Model file for the job. Use its own axes, mm. A direction names the side the tool comes from. Coordinates: 2 decimals unless noted, no trailing zeros. Write each loop counter-clockwise with the first axis right and the second up, starting at its lowest first coordinate (ties: lowest second). Pieces come first, ordered by that corner, then holes.
Q1. Band-saw the part on A-A, the plane z = 0. Write the cut outline in (x, y).
Q2. Drill centre lines: probe 1 along Y at (x, z) = (-3, 1); probe 2 along Z at (x, y) = (1.75, 4.25); probe 3 along X at (y, z) = (2.5, 0). Where is each one in solid material? Low to high.
Q3. Band-saw the part on C-C, the plane y = 2.25. Write the cut outline in (x, z).
Q4. Which spindle directions (+Z, -Z, +X, -X, +Y, -Y) get a long thin tool onto all of the face, cutting with end or side? Do faces 4 (the flat face through (-1.6, 4.4, -2)), 5 (the cylindrical face through (-3.593, 2.328, 1.869)). Say none if no direction does.
Q5. Band-saw the part on B-B, the plane x = 0. Write the cut outline in (y, z).
Q6. Pin check, flat tips, straight feed: P1, Ø0.8, axis at x = -1, z = -1.5, coming from the -Y side; P2, Ø1, axis at y = 0.5, z = -4, coming from the -X side; P3, Ø1.5, axis at x = 0.5, z = 0.5, coming from the +Y side. Stop position of each tip, or through.
Q7. Pull direction X, two halves, no side cores. Call faces 1 (the cylindrical face through (0.194, 0.246, 4.596)), 2 (the flat face through (0, 4.1, 0)), 3 (the flat face through (-1.6, 4.4, 2.1)): released by +X, released by -X, zero draft, split by the parting line, or undercut.
from build123d import *

# Parameters (mm, degrees)
SKETCH1_R                   = 4.05
BASE_EXTRUSION_DEPTH        = 4.2
SKETCH2_W                   = 3
SKETCH2_H                   = 4
WINDOW_DEPTH                = 0.1
WINDOW_BUMPS_DEPTH          = 0.2
WINDOW_BUMPS_CHAMFERS_SIZE  = 0.2
SKETCH3_R                   = 4.6
FLANGE_DEPTH                = 0.5
SKETCH5_W                   = 1.15
SKETCH5_H                   = 1
HORIZONTAL_FLANGE_TAB_DEPTH = 0.5
ROUNDS_AND_FILLETS_R        = 0.25
SKETCH4_R                   = 0.25
LEADS_DEPTH                 = 13.2


with BuildPart() as part:
    # Sketch1 → Base Extrusion (new body)
    with BuildSketch(Plane(origin=(0, 0, 0), x_dir=(1, 0, 0), z_dir=(0, 1, 0))):
        with Locations(Location((0, 0, 0), (0, 0, 270))):
            Circle(SKETCH1_R)
    extrude(amount=BASE_EXTRUSION_DEPTH)

    # Sketch2 → Window (cut)
    with BuildSketch(Plane(origin=(0, 4.2, 0), x_dir=(1, 0, 0), z_dir=(0, 1, 0))):
        Rectangle(SKETCH2_W, SKETCH2_H)
    extrude(amount=-WINDOW_DEPTH, mode=Mode.SUBTRACT)

    # Sketch6 → Window Bumps (add)
    with BuildSketch(Plane(origin=(0, 4.2, 0), x_dir=(1, 0, 0), z_dir=(0, 1, 0))):
        with BuildLine():
            Line((-0.75, 2), (-1.5, 1.25))
            ThreePointArc((-1.5, 1.25), (-2.030330086, 2.530330086), (-0.75, 2))
        make_face()
        with BuildLine():
            Line((0.75, 2), (1.5, 1.25))
            ThreePointArc((1.5, 1.25), (2.030330086, 2.530330086), (0.75, 2))
        make_face()
        with BuildLine():
            Line((1.5, -1.25), (0.75, -2))
            ThreePointArc((0.75, -2), (2.030330086, -2.530330086), (1.5, -1.25))
        make_face()
        with BuildLine():
            Line((-1.5, -1.25), (-0.75, -2))
            ThreePointArc((-0.75, -2), (-2.030330086, -2.530330086), (-1.5, -1.25))
        make_face()
    extrude(amount=WINDOW_BUMPS_DEPTH)

    # Window Bumps Chamfers
    window_bumps_chamfers_edges = [part.edges().sort_by_distance(p)[0] for p in [
        (-2.030330086, 4.4, 2.530330086),
        (2.030330086, 4.4, 2.530330086),
        (2.030330086, 4.4, -2.530330086),
        (-2.030330086, 4.4, -2.530330086),
        (-1.125, 4.4, 1.625),
        (1.125, 4.4, 1.625),
        (1.125, 4.4, -1.625),
        (-1.125, 4.4, -1.625),
    ]]
    chamfer(window_bumps_chamfers_edges, length=WINDOW_BUMPS_CHAMFERS_SIZE - 0.0001)  # a hair under: the kernel refuses the full size

    # Sketch3 → Flange (add)
    with BuildSketch(Plane.XZ):
        with Locations(Location((0, 0, 0), (0, 0, 270))):
            Circle(SKETCH3_R)
    extrude(amount=-FLANGE_DEPTH)

    # Sketch5 → Horizontal Flange Tab (add)
    with BuildSketch(Plane.XZ):
        with Locations((0, -5.063921012)):
            Rectangle(SKETCH5_W, SKETCH5_H)
    extrude(amount=-HORIZONTAL_FLANGE_TAB_DEPTH)

    # Rounds and Fillets
    rounds_and_fillets_edges = [part.edges().sort_by_distance(p)[0] for p in [
        (0, 4.2, -4.05),
        (0, 0.5, -4.05),
        (-0.575, 0.25, -5.563921012),
        (0.575, 0.25, -5.563921012),
    ]]
    fillet(rounds_and_fillets_edges, radius=ROUNDS_AND_FILLETS_R)

    # Sketch4 → Leads (add)
    with BuildSketch(Plane.XZ):
        with Locations(Location((-1.796051224, -1.796051224, 0), (0, 0, 90))):
            Circle(SKETCH4_R)
        with Locations(Location((1.796051224, 1.796051224, 0), (0, 0, 90))):
            Circle(SKETCH4_R)
        with Locations(Location((-1.796051224, 1.796051224, 0), (0, 0, 90))):
            Circle(SKETCH4_R)
    extrude(amount=LEADS_DEPTH)

    # Leads Trim
    split(bisect_by=Plane(origin=(0, -2, 0), x_dir=(1, 0, 0), z_dir=(0, 1, 0)), keep=Keep.TOP)


solid = part.part
Answer sheet:
1. outline: (-4.6, 0) - (4.6, 0) - (4.6, 0.5) - (4.3, 0.5) arc R0.25 cw to (4.05, 0.75) - (4.05, 3.95) arc R0.25 ccw to (3.8, 4.2) - (1.5, 4.2) - (1.5, 4.1) - (-1.5, 4.1) - (-1.5, 4.2) - (-3.8, 4.2) arc R0.25 ccw to (-4.05, 3.95) - (-4.05, 0.75) arc R0.25 cw to (-4.3, 0.5) - (-4.6, 0.5) - close
2. probe 1: y = 0 to 4.2
2. probe 2: z = -2.65 to -1.35, 1.35 to 2.65
2. probe 3: x = -4.05 to 4.05
3. outline: circle Ø8.1 at (0, 0)
4. face 4: +Z, -Z, +X, -X, +Y
4. face 5: +Y
5. outline: (0, -5.56) - (0.5, -5.56) - (0.5, -4.3) arc R0.25 cw to (0.75, -4.05) - (3.95, -4.05) arc R0.25 ccw to (4.2, -3.8) - (4.2, -2) - (4.1, -2) - (4.1, 2) - (4.2, 2) - (4.2, 3.8) arc R0.25 ccw to (3.95, 4.05) - (0.75, 4.05) arc R0.25 cw to (0.5, 4.3) - (0.5, 4.6) - (0, 4.6) - close
6. P1: stops at y = 0
6. P2: stops at x = -2.98
6. P3: stops at y = 4.1
7. face 1: split by the parting line
7. face 2: undercut
7. face 3: zero draft
